CAD build for the part. Positions are in the model's coordinates, mm. A direction names the side the tool comes from. Coordinates: 2 decimals unless noted, no trailing zeros. Loops run counter-clockwise (first coordinate to the right, second up) from the corner with the lowest first, then second, coordinate; pieces in that order, holes last. Notation, with made-up numbers: (-21, 27.5) -> (26, 27.5) arc R18 cw to (26, 46.5) -> close; hole circle Ø6 at (53.25, 0). An arc over 180 degrees is marked (long way). Answer as CSV lines item,"result". Start each with the question number.
from build123d import *

# Parameters (mm, degrees)
SKETCH1_W             = 42
SKETCH1_H             = 30
BOSS_EXTRUDE1_DEPTH   = 8
BOSS_EXTRUDE1_2_DEPTH = 8
BOSS_EXTRUDE2_DEPTH   = 30
SKETCH2_R             = 2.5
CUT_EXTRUDE1_DEPTH    = 8
SKETCH3_R             = 2.75
CUT_EXTRUDE2_DEPTH    = 10
SKETCH4_W             = 30
SKETCH4_H             = 100
CUT_EXTRUDE3_DEPTH    = 52


with BuildPart() as part:
    # Sketch1 → Boss-Extrude1 (new body)
    with BuildSketch(Plane.XY):
        with Locations((21, 133)):
            Rectangle(SKETCH1_W, SKETCH1_H)
    extrude(amount=BOSS_EXTRUDE1_DEPTH)



with BuildPart() as body_2:
    # Sketch1 → Boss-Extrude1 2 (new body)
    with BuildSketch(Plane.XY):
        with Locations((21, 15)):
            Rectangle(SKETCH1_W, SKETCH1_H)
    extrude(amount=BOSS_EXTRUDE1_2_DEPTH)


with BuildPart() as part_1:
    add(part.part)

    add(body_2.part)  # Boss-Extrude2 merges body 2
    # Sketch1<3> → Boss-Extrude2 (add)
    with BuildSketch(Plane.XY):
        Polygon((42, 30), (42, 0), (52, 0), (52, 148), (42, 148), (42, 118), align=None)
    extrude(amount=BOSS_EXTRUDE2_DEPTH)

    # Sketch2 → Cut-Extrude1 (cut)
    with BuildSketch(Plane.XY.offset(8)):
        with Locations((8, 133)):
            Circle(SKETCH2_R)
        with Locations((34, 133)):
            Circle(SKETCH2_R)
        with Locations((34, 15)):
            Circle(SKETCH2_R)
        with Locations((8, 15)):
            Circle(SKETCH2_R)
    extrude(amount=-CUT_EXTRUDE1_DEPTH, mode=Mode.SUBTRACT)

    # Sketch3 → Cut-Extrude2 (cut)
    with BuildSketch(Plane(origin=(52, 0, 0), x_dir=(0, 0, -1), z_dir=(1, 0, 0))):
        with Locations((-20, 138.3)):
            Circle(SKETCH3_R)
        with Locations((-20, 106.3)):
            Circle(SKETCH3_R)
        with Locations((-20, 41.2)):
            Circle(SKETCH3_R)
        with Locations((-20, 9.2)):
            Circle(SKETCH3_R)
    extrude(amount=-CUT_EXTRUDE2_DEPTH, mode=Mode.SUBTRACT)

    # Sketch4 → Cut-Extrude3 (cut)
    with BuildSketch(Plane(origin=(52, 0, 0), x_dir=(0, 0, -1), z_dir=(1, 0, 0))):
        with Locations((-15, 98)):
            Rectangle(SKETCH4_W, SKETCH4_H)
    extrude(amount=-CUT_EXTRUDE3_DEPTH, mode=Mode.SUBTRACT)


solid = part_1.part
Item 1: Which spindle directions (+Z, -Z, +X, -X, +Y, -Y) get a long thin tool onto all of the face, cutting with end or side? Do faces 5 (the face through (33.46, 12.56, 4.06)), 6 (the face through (21, 30, 4)). Say none if no direction does.
Item 2: Wall check: probe 1 along Y at (x, z) = (44.5, 20); probe 2 along Y at (x, z) = (8, 3.25); probe 3 along X at (y, z) = (16, 2.75). Give the ranges that are in metal, low to high.
Item 3: Saw through at A-A (z = 20). Write the cut outline in (x, y), plus the area to 3 significant figures.
Item 4: Flat gauge pins, fed straight in: pin 1 Ø3 at (x, y) = (23.5, 28) entering from +Z; pin 2 Ø2.5 at (x, z) = (23, 4.5) entering from +Y; pin 3 Ø4.5 at (y, z) = (41.2, 20) entering from +X. Where does each tip first touch, or does it go through?
Item 5: Two-plate mould, pull along Z, no slides. Class faces 1 (the face through (47.07, 9.321, 22.747)), 2 (the face through (47.07, 38.515, 20.596)), 3 (the face through (10.31, 14.04, 4.06)), 4 (the face through (21, 15, 8)): pulls with the +Z half, pulls with the -Z half, needs draft (parallel to the pull), parting line crosses it, or undercut.
Item 6: Saw through at B-B (y = 9.2). Write the cut outline in (x, z), plus the area to 3 significant figures.
Item 7: Saw through at C-C (x = 34). Write the cut outline in (y, z).
Item 8: Saw through at D-D (y = 15). Write the cut outline in (x, z).
Geometry check:
1,face 5,"+Z, -Z"
1,face 6,"+Z, -Z, -X, +Y"
2,probe 1,"0 to 6.45, 11.95 to 38.45, 43.95 to 48"
2,probe 2,"0 to 12.5, 17.5 to 30"
2,probe 3,"0 to 5.71, 10.29 to 31.71, 36.29 to 52"
3,outline,"(42, 0) -> (52, 0) -> (52, 6.45) -> (42, 6.45) -> close; (42, 11.95) -> (52, 11.95) -> (52, 38.45) -> (42, 38.45) -> close; (42, 43.95) -> (52, 43.95) -> (52, 48) -> (42, 48) -> close"
3,area,"370 mm2"
4,pin 1,"z = 8"
4,pin 2,"y = 30"
4,pin 3,"through"
5,face 1,"undercut"
5,face 2,"undercut"
5,face 3,"needs draft"
5,face 4,"pulls with the +Z half"
6,outline,"(0, 0) -> (52, 0) -> (52, 17.25) -> (42, 17.25) -> (42, 8) -> (0, 8) -> close; (42, 22.75) -> (52, 22.75) -> (52, 30) -> (42, 30) -> close"
6,area,"581 mm2"
7,outline,"(0, 0) -> (12.5, 0) -> (12.5, 8) -> (0, 8) -> close; (17.5, 0) -> (30, 0) -> (30, 8) -> (17.5, 8) -> close"
8,outline,"(0, 0) -> (5.5, 0) -> (5.5, 8) -> (0, 8) -> close; (10.5, 0) -> (31.5, 0) -> (31.5, 8) -> (10.5, 8) -> close; (36.5, 0) -> (52, 0) -> (52, 30) -> (42, 30) -> (42, 8) -> (36.5, 8) -> close"
